Geometry: final body of the model. Coordinates: model frame, mm. A direction names the side the tool comes from. Give positions to 0.01 mm unless a question says otherwise; leave off trailing zeros. Order: outer loops, then holes, each group sorted by start corner. A loop starts at its lowest first (then second) coordinate and runs counter-clockwise, first axis right, second up. Notation, with made-up numbers: (-18, 17) -> (23, 17) arc R16 ccw to (23, 32) -> close; hole circle Ø8 at (-37.75, 80.25). An arc over 180 degrees is marked (long way). Answer in a Markdown table with one row per item. Add a question column.
Q1. Cut plane C-C on x = -27.5. Return the cut outline in (y, z).
Q2. Cut plane A-A on z = 2.75. Return the cut outline in (x, y).
Q3. Pull-direction query (X, two-part tool) for faces 3 (the face through (-29, -6.126, 0)), 4 (the face through (-25, -23.126, 0)), 5 (the face through (-33.43, -3.62, 0.14)); classes: +X half, -X half, draft (parallel to the pull), parting line (faces both ways), or undercut.
Q4. Cut plane B-B on y = -17.5. Return the cut outline in (x, z).
Q5. Line query: line 1 along Y through (x, z) = (-27, -8.25); line 2 along X through (y, z) = (-16.5, -2.75); line 3 along X through (y, z) = (-19.75, -1.5). Output: solid intervals per line, ascending. Write a range as from..to.
Q6. Cut plane D-D on y = -8. Return the cut outline in (x, z), and give its area (3 significant figures).
Q7. Contact query for flat-ended pins moving along their axis: P1, Ø3.5, axis at x = -28, z = -2, coming from the -Y side; P2, Ø3, axis at x = -32, y = -12.5, coming from the -Z side. Output: stop coordinate, or through.
Q8. Set-up query: faces 1 (the face through (-25.836, -15, 0)), 2 (the face through (-32.4, -13, 10)). Return all of +Z, -Z, +X, -X, +Y, -Y with unobstructed straight access to the full face (end or side cutting, diameter ignored); none if empty.
from build123d import *

# Parameters (mm, degrees)
F1_DEPTH = 10
F2_SIZE  = 1


with BuildPart() as f1:
    # F0 (on Top) → F1 (new body, symmetric)
    with BuildSketch(Plane.XY):
        Polygon((-33.935995, -3.126303), (-33.935995, -23.126303), (-31.935995, -23.126303), (-32.435995, -6.126303), (-25.835995, -6.126303), (-25.835995, -23.126303), (-24.335995, -23.126303), (-24.335995, -3.126303), align=None)
    extrude(amount=F1_DEPTH, both=True)

    # F2
    f2_edges = [f1.edges().sort_by_distance(p)[0] for p in [
        (-33.935995, -3.126303, 0),
        (-24.335995, -3.126303, 0),
    ]]
    chamfer(f2_edges, length=F2_SIZE)


solid = f1.part
Completed:
| question | item | result |
|---|---|---|
| 1 | outline | (-6.13, -10) -> (-3.13, -10) -> (-3.13, 10) -> (-6.13, 10) -> close |
| 2 | outline | (-33.94, -23.13) -> (-31.94, -23.13) -> (-32.44, -6.13) -> (-25.84, -6.13) -> (-25.84, -23.13) -> (-24.34, -23.13) -> (-24.34, -4.13) -> (-25.34, -3.13) -> (-32.94, -3.13) -> (-33.94, -4.13) -> close |
| 3 | face 3 | undercut |
| 3 | face 4 | draft |
| 3 | face 5 | -X half |
| 4 | outline | (-33.94, -10) -> (-32.1, -10) -> (-32.1, 10) -> (-33.94, 10) -> close; (-25.84, -10) -> (-24.34, -10) -> (-24.34, 10) -> (-25.84, 10) -> close |
| 5 | line 1 | y = -6.13..-3.13 |
| 5 | line 2 | x = -33.94..-32.13, -25.84..-24.34 |
| 5 | line 3 | x = -33.94..-32.04, -25.84..-24.34 |
| 6 | outline | (-33.94, -10) -> (-32.38, -10) -> (-32.38, 10) -> (-33.94, 10) -> close; (-25.84, -10) -> (-24.34, -10) -> (-24.34, 10) -> (-25.84, 10) -> close |
| 6 | area | 61.1 mm² |
| 7 | P1 | stops at y = -6.13 |
| 7 | P2 | stops at z = -10 |
| 8 | face 1 | +Z, -Z, -Y |
| 8 | face 2 | +Z, +X, -X, +Y, -Y |
